Could you check a few things on this model? Use its own coordinates, in mm. Face numbers are marked on the shaded views. Round coordinates to 2 decimals unless told otherwise and drop trailing zeros. Write each loop counter-clockwise with the first axis right and the second up, starting at its lowest first coordinate (ties: lowest second). Pieces come first, ordered by that corner, then holes. Notation, with made-up numbers: (-16, 29) -> (33, 29) arc R15 cw to (33, 48) -> close; hole circle Ø3 at (-13, 78.5). An arc over 180 degrees is marked (long way). Answer in a Markdown table with one row per item.
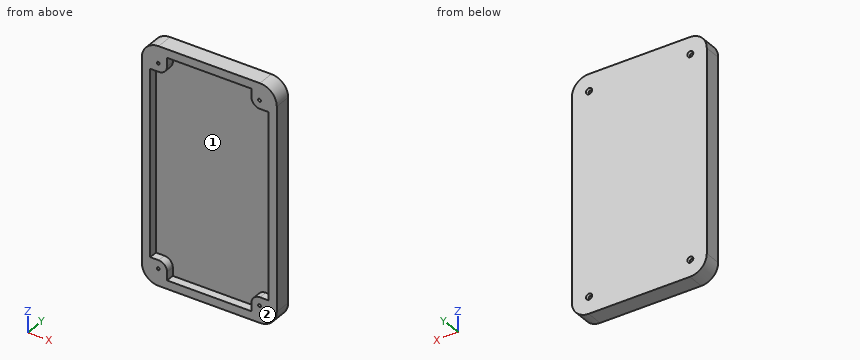
from build123d import *

# Parameters (mm, degrees)
SKETCH2_W                                            = 80
SKETCH2_H                                            = 140
BOSS_EXTRUDE1_DEPTH                                  = 10
SHELL2_T                                             = -5
BOSS_EXTRUDE4_REACH                                  = 83.24
FILLET3_R                                            = 10
CSK_FOR_M1_6_CROSS_RECESS_FLAT_HEAD_SCRE_D           = 1.7
CSK_FOR_M1_6_CROSS_RECESS_FLAT_HEAD_SCRE_CSINK_D     = 3.6
CSK_FOR_M1_6_CROSS_RECESS_FLAT_HEAD_SCRE_CSINK_ANGLE = 90


with BuildPart() as part:
    # Sketch2 → Boss-Extrude1 (new body)
    with BuildSketch(Plane(origin=(0, 0, 0), x_dir=(1, 0, 0), z_dir=(0, 1, 0))):
        Rectangle(SKETCH2_W, SKETCH2_H)
    extrude(amount=BOSS_EXTRUDE1_DEPTH)

    # Shell2
    shell2_openings = [part.faces().sort_by_distance(p)[0] for p in [
        (0, 0, 0),
    ]]
    offset(amount=SHELL2_T, openings=shell2_openings, kind=Kind.INTERSECTION)

    # Sketch6 → Boss-Extrude4 (add, up to next)
    with BuildSketch(Plane.XZ, mode=Mode.PRIVATE) as boss_extrude4_sk1:
        with BuildLine():
            Line((-30, 55), (-35, 55))
            Line((-35, 55), (-35, 65))
            Line((-35, 65), (-25, 65))
            Line((-25, 65), (-25, 60))
            ThreePointArc((-25, 60), (-26.464466094, 56.464466094), (-30, 55))
        make_face()
    boss_extrude4_tool1 = extrude(boss_extrude4_sk1.sketch, amount=-BOSS_EXTRUDE4_REACH, mode=Mode.PRIVATE) - part.part
    # Sketch6 → Boss-Extrude4 (add, up to next)
    with BuildSketch(Plane.XZ, mode=Mode.PRIVATE) as boss_extrude4_sk2:
        with BuildLine():
            Line((25, 60), (25, 65))
            Line((25, 65), (35, 65))
            Line((35, 65), (35, 55))
            Line((35, 55), (30, 55))
            ThreePointArc((30, 55), (26.464466094, 56.464466094), (25, 60))
        make_face()
    boss_extrude4_tool2 = extrude(boss_extrude4_sk2.sketch, amount=-BOSS_EXTRUDE4_REACH, mode=Mode.PRIVATE) - part.part
    # Sketch6 → Boss-Extrude4 (add, up to next)
    with BuildSketch(Plane.XZ, mode=Mode.PRIVATE) as boss_extrude4_sk3:
        with BuildLine():
            Line((30, -55), (35, -55))
            Line((35, -55), (35, -65))
            Line((35, -65), (25, -65))
            Line((25, -65), (25, -60))
            ThreePointArc((25, -60), (26.464466094, -56.464466094), (30, -55))
        make_face()
    boss_extrude4_tool3 = extrude(boss_extrude4_sk3.sketch, amount=-BOSS_EXTRUDE4_REACH, mode=Mode.PRIVATE) - part.part
    # Sketch6 → Boss-Extrude4 (add, up to next)
    with BuildSketch(Plane.XZ, mode=Mode.PRIVATE) as boss_extrude4_sk4:
        with BuildLine():
            Line((-25, -60), (-25, -65))
            Line((-25, -65), (-35, -65))
            Line((-35, -65), (-35, -55))
            Line((-35, -55), (-30, -55))
            ThreePointArc((-30, -55), (-26.464466094, -56.464466094), (-25, -60))
        make_face()
    boss_extrude4_tool4 = extrude(boss_extrude4_sk4.sketch, amount=-BOSS_EXTRUDE4_REACH, mode=Mode.PRIVATE) - part.part
    add(boss_extrude4_tool1.solids().sort_by_distance((-30.220144, 0, 60.220144))[0])
    add(boss_extrude4_tool2.solids().sort_by_distance((30.220144, 0, 60.220144))[0])
    add(boss_extrude4_tool3.solids().sort_by_distance((30.220144, 0, -60.220144))[0])
    add(boss_extrude4_tool4.solids().sort_by_distance((-30.220144, 0, -60.220144))[0])

    # Fillet3
    fillet3_edges = [part.edges().sort_by_distance(p)[0] for p in [
        (40, 5, 70),
        (-40, 5, 70),
        (-40, 5, -70),
        (40, 5, -70),
    ]]
    fillet(fillet3_edges, radius=FILLET3_R)

    # CSK for M1.6 Cross Recess Flat Head Screw1 (through all)
    with Locations(Plane(origin=(0, 10, 0), x_dir=(1, 0, 0), z_dir=(0, 1, 0))):
        with Locations((-30.216332876, 60.028429813), (29.772350977, 60.028429813), (29.772350977, -59.957909435), (-30.216332876, -59.957909435)):
            CounterSinkHole(CSK_FOR_M1_6_CROSS_RECESS_FLAT_HEAD_SCRE_D / 2, CSK_FOR_M1_6_CROSS_RECESS_FLAT_HEAD_SCRE_CSINK_D / 2, counter_sink_angle=CSK_FOR_M1_6_CROSS_RECESS_FLAT_HEAD_SCRE_CSINK_ANGLE)


solid = part.part
1) Imagine slicing it at B-B, the plane x = 33. Please give me the cut outline in (y, z), plus the area to 3 significant figures.
Findings:
| item | result |
|---|---|
| outline | (0, -69.54) -> (10, -69.54) -> (10, 69.54) -> (0, 69.54) -> (0, 55) -> (5, 55) -> (5, -55) -> (0, -55) -> close |
| area | 841 mm^2 |
2) Please list where these lines run through material, in increasing order: line 1 (X direction, y = 1.5, z = -3.5); line 2 (Z direction, x = -18, y = 1.75); line 3 (Y direction, x = 4.5, z = 60.5).
Findings:
| item | result |
|---|---|
| line 1 | x = -40 to -35, 35 to 40 |
| line 2 | z = -70 to -65, 65 to 70 |
| line 3 | y = 5 to 10 |
3) Imagine slicing it at A-A, the plane z = 33.5. Please give me the cut outline in (x, y), plus the area to 3 significant figures.
Findings:
| item | result |
|---|---|
| outline | (-40, 0) -> (-35, 0) -> (-35, 5) -> (35, 5) -> (35, 0) -> (40, 0) -> (40, 10) -> (-40, 10) -> close |
| area | 450 mm^2 |
4) For pin 1 (5.5 mm diameter, centred on x = -31.5, y = 1.5, fed in from +Z); pin 2 (5.5 mm diameter, centred on x = 33.5, y = 3.5, fed in from -Z); pin 3 (2 mm diameter, centred on x = -30.22, z = 59.96, fed in from +Y); pin 4 (2.5 mm diameter, centred on y = 3.5, z = 61.5, fed in from -X), each with a flat end and sliding along its axis, tell me the tip position at first contact or that it passes through.
Findings:
| item | result |
|---|---|
| pin 1 | stops at z = 70 |
| pin 2 | stops at z = -69.97 |
| pin 3 | stops at y = 9.2 |
| pin 4 | stops at x = -40 |
5) Thinking about a two-plate mould opening in X: for the marked faces 1 and 2, which applies, +X half, -X half, draft (parallel to the pull), parting line (faces both ways), or undercut?
Findings:
| item | result |
|---|---|
| face 1 | undercut |
| face 2 | draft |
